```python
from build123d import *

# Parameters (mm, degrees)
SKETCH_1_W         = 12
SKETCH_1_H         = 18
SKETCH_1_W_2       = 8
SKETCH_1_H_2       = 15
EXTRUDE_1_DEPTH    = 8
SKETCH_1_3_W       = 8
SKETCH_1_3_H       = 7.5
EXTRUDE_2_DEPTH    = 1.5
HOLE_WIZARD_M3_1_D = 2.5
FILLET_2_R         = 4
FILLET_3_R         = 2


with BuildPart() as part:
    # 草图1 → 凸台-拉伸1 (new body)
    with BuildSketch(Plane.XY):
        with Locations((4, 7)):
            Rectangle(SKETCH_1_W, SKETCH_1_H)
        with Locations((4, 7.5)):
            Rectangle(SKETCH_1_W_2, SKETCH_1_H_2, mode=Mode.SUBTRACT)
    extrude(amount=EXTRUDE_1_DEPTH)

    # 草图1<3> → 凸台-拉伸2 (add)
    with BuildSketch(Plane.XY):
        with Locations((4, 3.75)):
            Rectangle(SKETCH_1_3_W, SKETCH_1_3_H)
    extrude(amount=EXTRUDE_2_DEPTH)

    # M3 螺纹孔1 (through all)
    with Locations(Plane(origin=(10, 0, 0), x_dir=(0, 0, -1), z_dir=(1, 0, 0))):
        with Locations((-4.5, 2.5)):
            Hole(HOLE_WIZARD_M3_1_D / 2)

    # 圆角2
    fillet_2_edges = [part.edges().sort_by_distance(p)[0] for p in [
        (-2, 16, 4),
        (10, 16, 4),
    ]]
    fillet(fillet_2_edges, radius=FILLET_2_R)

    # 圆角3
    fillet_3_edges = [part.edges().sort_by_distance(p)[0] for p in [
        (10, -2, 4),
        (-2, -2, 4),
    ]]
    fillet(fillet_3_edges, radius=FILLET_3_R)


solid = part.part
```
Could you check a few things on this model? Use its own coordinates, in mm. A direction names the side the tool comes from. Round coordinates to 2 decimals unless told otherwise and drop trailing zeros. Loops run counter-clockwise (first coordinate to the right, second up) from the corner with the lowest first, then second, coordinate; pieces in that order, holes last. Notation, with made-up numbers: M 33.25,62 L 37.25,62 A20 ccw 37.25,93 Z; hole C -0.5,-25 d5. An arc over 180 degrees is marked long. Answer as CSV lines item,"result".
1) Which directions (+Z, -Z, +X, -X, +Y, -Y) give clear straight access to the entire face, cutting with the end or side of a thin tool? Please do faces 4 (the flat face through (4, 15, 4)), 5 (the flat face through (10, 6, 4)), 6 (the flat face through (0, 7, 4)).
From the geometry:
face 4,"+Z, -Z"
face 5,"+Z, -Z, +X, +Y, -Y"
face 6,"+Z"
2) If I drill on probe 1 along X at (y, z) = (10.5, 5.75); probe 2 along Y at (x, z) = (5, 6.5); probe 3 along Y at (x, z) = (5.5, 1), over which ranges is the centre line in solid material (lowest first)?
From the geometry:
probe 1,"-2 to 0, 8 to 10"
probe 2,"-2 to 0, 15 to 16"
probe 3,"-2 to 7.5, 15 to 16"
3) We'd pull the mould along Y, two halves only. Please class faces 1 (the cylindrical face through (-1.43, -1.4, 4.06)), 2 (the flat face through (4, 4, 1.5)), 3 (the cylindrical face through (8.859, 14.797, 4.056)): released by +Y, released by -Y, zero draft, split by the parting line, or undercut.
From the geometry:
face 1,"released by -Y"
face 2,"undercut"
face 3,"released by +Y"
4) Imagine slicing it at D-D on z = 3.5. List the corners of the cut face in (x, y) for me, and give its area (3 significant figures).
From the geometry:
outline,"M -2,0 A2 ccw 0,-2 L 8,-2 A2 ccw 10,0 L 10,1.75 L 8,1.75 L 8,0 L 0,0 L 0,1.75 L -2,1.75 Z; M -2,3.25 L 0,3.25 L 0,15 L 8,15 L 8,3.25 L 10,3.25 L 10,12 A4 ccw 6,16 L 2,16 A4 ccw -2,12 Z"
area,"81.4 mm^2"
5) Imagine slicing it at B-B on x = 5.25. List the corners of the cut face in (y, z) for me, and give its area (4 significant figures).
From the geometry:
outline,"M -2,0 L 7.5,0 L 7.5,1.5 L 0,1.5 L 0,8 L -2,8 Z; M 15,0 L 16,0 L 16,8 L 15,8 Z"
area,"35.25 mm^2"
6) For pin 1 Ø3 at (y, z) = (2.5, 4.5) entering from -X; pin 2 Ø2 at (y, z) = (2.5, 4.5) entering from -X, each with a flat end and sliding along its axis, tell me the tip position at first contact or that it passes through.
From the geometry:
pin 1,"x = -2"
pin 2,"through"
7) Imagine slicing it at C-C on y = 10.5. List the corners of the cut face in (x, z) for me, and give its area (3 significant figures).
From the geometry:
outline,"M -2,0 L 0,0 L 0,8 L -2,8 Z; M 8,0 L 10,0 L 10,8 L 8,8 Z"
area,"32.0 mm^2"
8) Imagine slicing it at A-A on z = 6.5. List the corners of the cut face in (x, y) for me.
From the geometry:
outline,"M -2,0 A2 ccw 0,-2 L 8,-2 A2 ccw 10,0 L 10,12 A4 ccw 6,16 L 2,16 A4 ccw -2,12 Z; hole M 0,0 L 8,0 L 8,15 L 0,15 Z"
